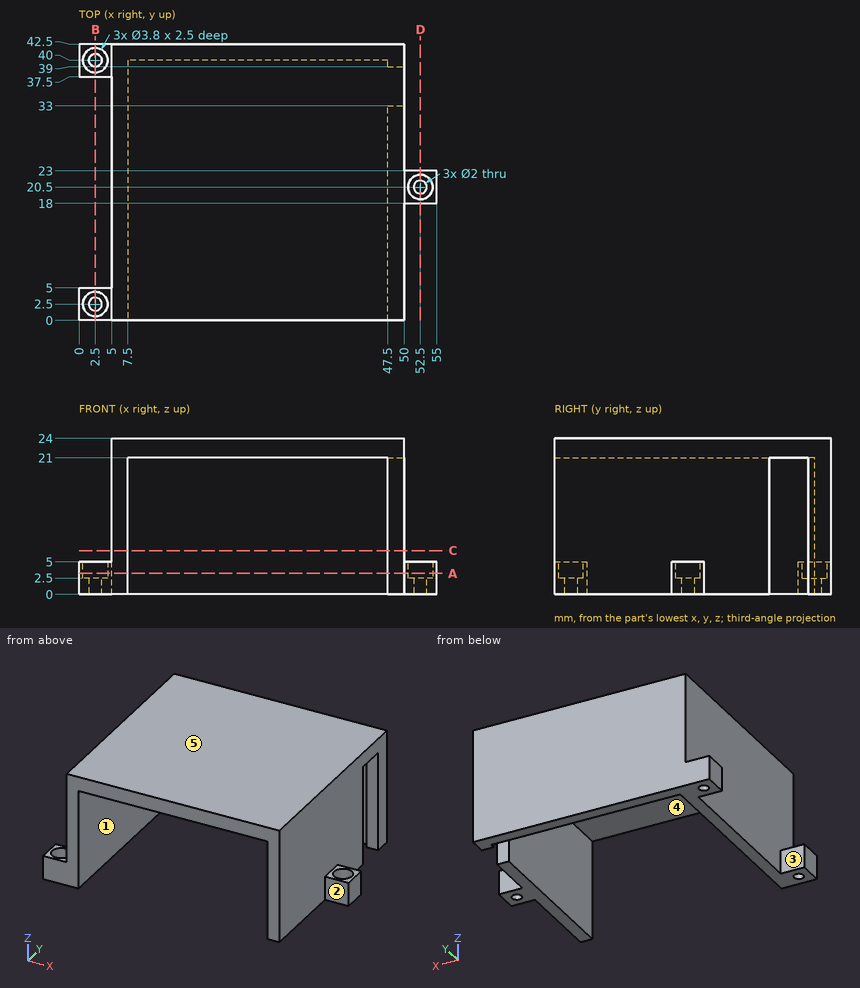
Print and shaded views of the part. All mm, measured from the part's lowest x, y and z. A direction names the side the tool comes from. Give positions to 0.01 mm unless a question says otherwise; leave off trailing zeros. Order: outer loops, then holes, each group sorted by start corner. A loop starts at its lowest first (then second) coordinate and runs counter-clockwise, first axis right, second up. Notation, with made-up numbers: M 13.25,47 L 42.25,47 A4 ccw 42.25,54 Z; hole C 62,65 d2. An arc over 180 degrees is marked long. Use one line per item in the form item = value.
Q1. Which spindle directions (+Z, -Z, +X, -X, +Y, -Y) get a long thin tool onto all of the face, cutting with end or side? Do the marked faces 1, 2 and 3. Say none if no direction does.
Conclusion:
face_1 = -Z, -Y
face_2 = +Z, -Z, +X, -Y
face_3 = +Z, -Z, -X
Q2. Slice it at C-C, the plane z = 6.75. Write the cut outline in (x, y).
Conclusion:
outline = M 5,0 L 7.5,0 L 7.5,40 L 47.5,40 L 47.5,39 L 50,39 L 50,42.5 L 5,42.5 Z; M 47.5,0 L 50,0 L 50,33 L 47.5,33 Z
Q3. Slice it at A-A, the plane z = 3.25. Write the cut outline in (x, y), and give its area (3 significant figures).
Conclusion:
outline = M 0,0 L 7.5,0 L 7.5,40 L 47.5,40 L 47.5,39 L 50,39 L 50,42.5 L 0,42.5 L 0,37.5 L 5,37.5 L 5,5 L 0,5 Z; M 47.5,0 L 50,0 L 50,18 L 55,18 L 55,23 L 50,23 L 50,33 L 47.5,33 Z; hole C 2.5,2.5 d3.8; hole C 2.5,40 d3.8; hole C 52.5,20.5 d3.8
area = 338 mm2
Q4. Slice it at D-D, the plane x = 52.5. Write the cut outline in (y, z).
Conclusion:
outline = M 18,0 L 19.5,0 L 19.5,2.5 L 18.6,2.5 L 18.6,5 L 18,5 Z; M 21.5,0 L 23,0 L 23,5 L 22.4,5 L 22.4,2.5 L 21.5,2.5 Z
Q5. Pin check, flat tips, straight feed: P1, Ø8, axis at x = 17, z = 3, coming from the -Y side; P2, Ø1.5, axis at x = 14.5, y = 36, coming from the -Z side; P3, Ø2, axis at y = 13.5, z = 19, coming from the -X side. Stop position of each tip, or through.
Conclusion:
P1 = 40
P2 = 21
P3 = 5
Q6. Pull direction X, two halves, no side cores. Call the marked faces 4 and 5: released by +X, released by -X, zero draft, split by the parting line, or undercut.
Conclusion:
face_4 = undercut
face_5 = zero draft
Q7. Wall check: probe 1 along X at (y, z) = (2.5, 4.35); probe 2 along Y at (x, z) = (2.5, 0.8); probe 3 along X at (y, z) = (28.5, 20.25). Give the ranges that are in metal, low to high.
Conclusion:
probe_1 = 0 to 0.6, 4.4 to 7.5, 47.5 to 50
probe_2 = 0 to 1.5, 3.5 to 5, 37.5 to 39, 41 to 42.5
probe_3 = 5 to 7.5, 47.5 to 50
Q8. Slice it at B-B, the plane x = 2.5. Write the cut outline in (y, z), and give its area (3 significant figures).
Conclusion:
outline = M 0,0 L 1.5,0 L 1.5,2.5 L 0.6,2.5 L 0.6,5 L 0,5 Z; M 3.5,0 L 5,0 L 5,5 L 4.4,5 L 4.4,2.5 L 3.5,2.5 Z; M 37.5,0 L 39,0 L 39,2.5 L 38.1,2.5 L 38.1,5 L 37.5,5 Z; M 41,0 L 42.5,0 L 42.5,5 L 41.9,5 L 41.9,2.5 L 41,2.5 Z
area = 21.0 mm2
